Autodesk Inventor part; units mm, degrees
ref_plane "YZ Plane" through (0, 0, 0) normal (1, 0, 0) x (0, 1, 0)
ref_plane "XZ Plane" through (0, 0, 0) normal (0, 1, 0) x (-1, 0, 0)
ref_plane "XY Plane" through (0, 0, 0) normal (0, 0, 1) x (1, 0, 0)
sketch "草圖1" plane through (0, 0, 0) normal (0, 1, 0) x (-1, 0, 0)
  circle A0 centre (0, 0) radius 20
  line L0 (0, 20) -> (0, -20)
  dimension "d0" = 40
revolve "迴轉1" add sketch "草圖1" angle 180 about axis through (0, 0, 20) along (0, 0, -1) picked at (-3.0982, -5.903) contours L0 A0
sketch "草圖2" plane through (0, 0, 0) normal (0, 0, 1) x (1, 0, 0)
  line L0 (20, 0) -> (-20, 0)
  arc A0 (-20, 0) -> (20, 0) centre (0, 0) ccw
  arc A1 (-20, 0) -> (20, 0) centre (0, 0) ccw
  arc A2 (-19, 0) -> (19, 0) centre (0, 0) ccw
  line L1 (-19, 0) -> (-20, 0)
  line L2 (19, 0) -> (20, 0)
  dimension "d2" = 1
extrude "擠出1" cut sketch "草圖2" along normal mid plane 1 contours A0 L0 A2
sketch "草圖3" plane through (0, 0, 0) normal (1, 0, 0) x (0, 1, 0)
  line L0 (0, 0.5) -> (0, 20)
  line L1 (0, -20) -> (0, -0.5)
  arc A0 (0, 19) -> (0, -19) centre (0, 0) ccw
  arc A1 (0, 20) -> (0, -20) centre (0, 0) ccw
  line L2 (0, 20) -> (0, 19)
  line L3 (0, -20) -> (0, -19)
  dimension "d5" = 1
extrude "擠出2" cut sketch "草圖3" along normal mid plane 1
properties part number "屋2 base"
Can you work these out from the model? Positions are in its coordinate system, mm. A direction names the side the tool comes from. Give positions to 0.01 mm unless a question says otherwise; leave off trailing zeros. Order: outer loops, then holes, each group sorted by start corner. A loop starts at its lowest first (then second) coordinate and runs counter-clockwise, first axis right, second up. Notation, with made-up numbers: M -20.5,65 L -1.5,65 A18 cw -1.5,78 Z; hole C -27.5,-16.75 d10. An arc over 180 degrees is marked long. Use one line per item in the form item = value.
Item 1: Thinking about a two-plate mould opening in X: for faces 4 (the cylindrical face through (-13.29, -13.58, -0.01)), 5 (the cylindrical face through (13.58, -13.29, -0.01)), 6 (the flat face through (-0.5, -12, 15)), 7 (the flat face through (0.5, -12, 15)), which applies, pulls with the +X half, pulls with the -X half, needs draft (parallel to the pull), parting line crosses it, or undercut?
Values follow:
face_4 = pulls with the -X half
face_5 = pulls with the +X half
face_6 = undercut
face_7 = undercut
Item 2: If we section it at A-A, the plane y = -8.75: Write out the boundary of the cut face in (x, z), and give its area (3 significant figures).
Values follow:
outline = M -17.98,-0.5 A17.98 ccw -0.5,-17.98 L -0.5,-16.87 L 0.5,-16.87 L 0.5,-17.98 A17.98 ccw 17.98,-0.5 L 16.87,-0.5 L 16.87,0.5 L 17.98,0.5 A17.98 ccw 0.5,17.98 L 0.5,16.87 L -0.5,16.87 L -0.5,17.98 A17.98 ccw -17.98,0.5 L -16.87,0.5 L -16.87,-0.5 Z
area = 1,010 mm^2
Item 3: If we section it at D-D, the plane y = -14.5: Write out the boundary of the cut face in (x, z), and give its area (3 significant figures).
Values follow:
outline = M -13.77,-0.5 A13.77 ccw -0.5,-13.77 L -0.5,-12.28 L 0.5,-12.28 L 0.5,-13.77 A13.77 ccw 13.77,-0.5 L 12.28,-0.5 L 12.28,0.5 L 13.77,0.5 A13.77 ccw 0.5,13.77 L 0.5,12.28 L -0.5,12.28 L -0.5,13.77 A13.77 ccw -13.77,0.5 L -12.28,0.5 L -12.28,-0.5 Z
area = 590 mm^2
Item 4: If I drill on line 1 along Y through (x, z) = (-7.5, 6.5); line 2 along Z through (x, y) = (-6, -1.75); line 3 along Z through (x, y) = (-7.5, -15), over which ranges is the centre line in solid material (lowest first)? Write a range as [from, to].
Values follow:
line_1 = [-17.36, 0]
line_2 = [-19, 19]
line_3 = [-10.9, 10.9]
Item 5: For faces 1 (the flat face through (-15, -12, 0.5)), 2 (the flat face through (0, 0, 0)), 3 (the flat face through (14, -14, 0.5)), which set-ups out of +Z, -Z, +X, -X, +Y, -Y let a thin tool reach every point of the face, with its end or its side?
Values follow:
face_1 = -X, -Y
face_2 = +Z, -Z, +X, -X, +Y
face_3 = +X, -Y
Item 6: If we section it at B-B, the plane z = -11: Write out the boundary of the cut face in (x, y).
Values follow:
outline = M -16.7,0 A16.7 ccw -0.5,-16.7 L -0.5,-15.49 L 0.5,-15.49 L 0.5,-16.7 A16.7 ccw 16.7,0 Z
Item 7: Will these pins go through, and if not, where does the flat tip stop? pin 1 Ø8 at (x, z) = (-5, 13) entering from +Y; pin 2 Ø9.5 at (x, y) = (9, -13) entering from +Z; pin 3 Ø9.5 at (y, z) = (-12.5, 10) entering from -X; pin 4 Ø3 at (x, z) = (-5, 6) entering from -Y.
Values follow:
pin_1 = 0
pin_2 = 16.66
pin_3 = -16.53
pin_4 = -18.98
Item 8: If we section it at C-C, the plane x = 13.5: Write out the boundary of the cut face in (y, z), and give its area (3 significant figures).
Values follow:
outline = M -14.75,-0.5 A14.76 ccw 0,-14.76 L 0,14.76 A14.76 ccw -14.75,0.5 L -13.37,0.5 L -13.37,-0.5 Z
area = 341 mm^2
